Check sheet for the modelled part. Datum: model origin and axes. Units: mm. Face numbers are marked on the shaded views. Coordinates: 2 decimals unless noted, no trailing zeros. Order: outer loops, then holes, each group sorted by start corner. A loop starts at its lowest first (then second) coordinate and runs counter-clockwise, first axis right, second up.
1. Cross-section at B-B (x = -90). Enter the section's corners in (y, z).
2. Gauge pin test, flat ends, axial feed: pin 1 Ø11 at (x, z) = (82.5, -45) entering from +Y; pin 2 Ø17.5 at (x, z) = (-17, -28) entering from +Y; pin 3 Ø1 at (y, z) = (1.5, -0.5) entering from -X. Record the tip position at first contact, or that the pin passes through.
3. Cross-section at A-A (z = 21). Enter the section's corners in (x, y).
4. Draft check along Z on the marked faces 1 and 2. Enter one of: released by +Z, released by -Z, zero draft, split by the parting line, or undercut.
5. Thickness scan on line 1 (Z direction, x = 65.5, y = 1.75); line 2 (X direction, y = 2, z = -44); line 3 (X direction, y = 9, z = 19.5). Record the ranges inside material, lowest first.
```python
from build123d import *

# Parameters (mm, degrees)
SKETCH1_W    = 203.2
SKETCH1_H    = 124.46
SKETCH1_W_2  = 44.45
SKETCH1_H_2  = 22.86
SKETCH1_H_3  = 21.59
SKETCH1_W_3  = 50.8
SKETCH1_W_4  = 97.79
TRAY_DEPTH   = 10.16
SKETCH3_W    = 203.2
SKETCH3_H    = 124.46
BASE_DEPTH   = 2.54
HANDLE_DEPTH = 124.46


with BuildPart() as part:
    # Sketch1 → tray (new body)
    with BuildSketch(Plane(origin=(0, 0, 0), x_dir=(1, 0, 0), z_dir=(0, 1, 0))):
        Rectangle(SKETCH1_W, SKETCH1_H)
        with Locations((76.835, -48.26)):
            Rectangle(SKETCH1_W_2, SKETCH1_H_2, mode=Mode.SUBTRACT)
        with Locations((76.835, 48.895)):
            Rectangle(SKETCH1_W_2, SKETCH1_H_3, mode=Mode.SUBTRACT)
        with Locations((-73.66, -48.26)):
            Rectangle(SKETCH1_W_3, SKETCH1_H_2, mode=Mode.SUBTRACT)
        with Locations((-73.66, 48.895)):
            Rectangle(SKETCH1_W_3, SKETCH1_H_3, mode=Mode.SUBTRACT)
        with Locations((-73.66, 24.765)):
            Rectangle(SKETCH1_W_3, SKETCH1_H_3, mode=Mode.SUBTRACT)
        with Locations((-73.66, 0.635)):
            Rectangle(SKETCH1_W_3, SKETCH1_H_3, mode=Mode.SUBTRACT)
        with Locations((-73.66, -23.495)):
            Rectangle(SKETCH1_W_3, SKETCH1_H_3, mode=Mode.SUBTRACT)
        with Locations((-20.32, 48.895)):
            Rectangle(SKETCH1_W_3, SKETCH1_H_3, mode=Mode.SUBTRACT)
        with Locations((29.845, 48.895)):
            Rectangle(SKETCH1_W_2, SKETCH1_H_3, mode=Mode.SUBTRACT)
        with Locations((-20.32, -23.495)):
            Rectangle(SKETCH1_W_3, SKETCH1_H_3, mode=Mode.SUBTRACT)
        with Locations((29.845, -23.495)):
            Rectangle(SKETCH1_W_2, SKETCH1_H_3, mode=Mode.SUBTRACT)
        with Locations((29.845, 24.765)):
            Rectangle(SKETCH1_W_2, SKETCH1_H_3, mode=Mode.SUBTRACT)
        with Locations((-20.32, 24.765)):
            Rectangle(SKETCH1_W_3, SKETCH1_H_3, mode=Mode.SUBTRACT)
        with Locations((3.175, 0.635)):
            Rectangle(SKETCH1_W_4, SKETCH1_H_3, mode=Mode.SUBTRACT)
        with Locations((3.175, -48.26)):
            Rectangle(SKETCH1_W_4, SKETCH1_H_2, mode=Mode.SUBTRACT)
        with Locations((76.835, -23.495)):
            Rectangle(SKETCH1_W_2, SKETCH1_H_3, mode=Mode.SUBTRACT)
        with Locations((76.835, 0.635)):
            Rectangle(SKETCH1_W_2, SKETCH1_H_3, mode=Mode.SUBTRACT)
        with Locations((76.835, 24.765)):
            Rectangle(SKETCH1_W_2, SKETCH1_H_3, mode=Mode.SUBTRACT)
    extrude(amount=TRAY_DEPTH)

    # Sketch3 → base (add)
    with BuildSketch(Plane(origin=(0, 0, 0), x_dir=(-1, 0, 0), z_dir=(0, -1, 0))):
        Rectangle(SKETCH3_W, SKETCH3_H)
    extrude(amount=BASE_DEPTH)

    # Sketch4 → handle (add)
    with BuildSketch(Plane.XY.offset(62.23)):
        with BuildLine():
            Line((-101.6, -2.54), (-101.6, 10.16))
            Line((-101.6, 10.16), (-109.22, 10.16))
            Line((-109.22, 10.16), (-109.22, 5.08))
            Line((-109.22, 5.08), (-106.68, 5.08))
            Line((-106.68, 5.08), (-106.68, 6.35))
            ThreePointArc((-106.68, 6.35), (-104.883948776, 5.606051224), (-104.14, 3.81))
            Line((-104.14, 3.81), (-104.14, -2.54))
            Line((-104.14, -2.54), (-101.6, -2.54))
        make_face()
        with BuildLine():
            Line((101.6, -2.54), (104.14, -2.54))
            Line((104.14, -2.54), (104.14, 3.81))
            ThreePointArc((104.14, 3.81), (104.883948776, 5.606051224), (106.68, 6.35))
            Line((106.68, 6.35), (106.68, 5.08))
            Line((106.68, 5.08), (109.22, 5.08))
            Line((109.22, 5.08), (109.22, 10.16))
            Line((109.22, 10.16), (101.6, 10.16))
            Line((101.6, 10.16), (101.6, -2.54))
        make_face()
    extrude(amount=-HANDLE_DEPTH)


solid = part.part
```
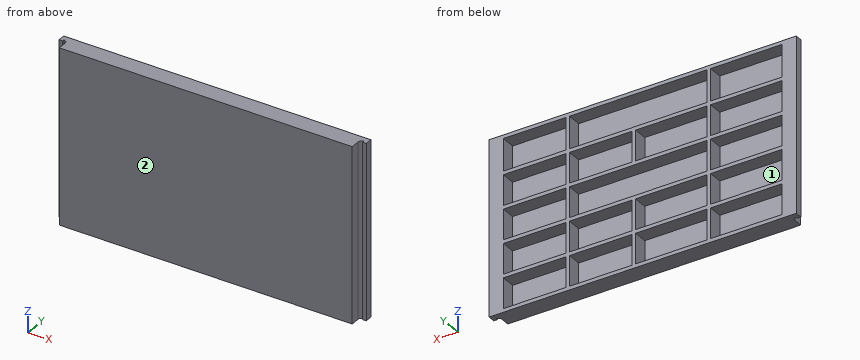
Data:
1. outline: (-2.54, -62.23) - (10.16, -62.23) - (10.16, -59.69) - (0, -59.69) - (0, -38.1) - (10.16, -38.1) - (10.16, -35.56) - (0, -35.56) - (0, -13.97) - (10.16, -13.97) - (10.16, -11.43) - (0, -11.43) - (0, 10.16) - (10.16, 10.16) - (10.16, 12.7) - (0, 12.7) - (0, 34.29) - (10.16, 34.29) - (10.16, 36.83) - (0, 36.83) - (0, 59.69) - (10.16, 59.69) - (10.16, 62.23) - (-2.54, 62.23) - close
2. pin 1: stops at y = 0
2. pin 2: stops at y = 10.16
2. pin 3: stops at x = -104.14
3. outline: (-109.22, 5.08) - (-106.68, 5.08) - (-106.68, 6.35) arc R2.54 cw to (-104.14, 3.81) - (-104.14, -2.54) - (104.14, -2.54) - (104.14, 3.81) arc R2.54 cw to (106.68, 6.35) - (106.68, 5.08) - (109.22, 5.08) - (109.22, 10.16) - (99.06, 10.16) - (99.06, 0) - (54.61, 0) - (54.61, 10.16) - (52.07, 10.16) - (52.07, 0) - (7.62, 0) - (7.62, 10.16) - (5.08, 10.16) - (5.08, 0) - (-45.72, 0) - (-45.72, 10.16) - (-48.26, 10.16) - (-48.26, 0) - (-99.06, 0) - (-99.06, 10.16) - (-109.22, 10.16) - close
4. face 1: undercut
4. face 2: zero draft
5. line 1: z = -62.23 to -59.69, -38.1 to -35.56, -13.97 to -11.43, 10.16 to 12.7, 34.29 to 36.83, 59.69 to 62.23
5. line 2: x = -104.14 to -99.06, -48.26 to -45.72, 5.08 to 7.62, 52.07 to 54.61, 99.06 to 104.14
5. line 3: x = -109.22 to -99.06, -48.26 to -45.72, 5.08 to 7.62, 52.07 to 54.61, 99.06 to 109.22
